Verification items for the finished model (mm, model axes). A direction names the side the tool comes from. Round coordinates to 2 decimals unless told otherwise and drop trailing zeros. Loops run counter-clockwise (first coordinate to the right, second up) from the corner with the lowest first, then second, coordinate; pieces in that order, holes last. Notation, with made-up numbers: (57.25, 70.5) - (104.25, 70.5) arc R18 cw to (104.25, 98.5) - close; hole circle Ø8 at (7.25, 76). An arc over 180 degrees is marked (long way). Use a Markdown table: item, result. Add a question column.
```python
from build123d import *

# Parameters (mm, degrees)
SKETCH1_W                    = 1165
SKETCH1_H                    = 40
BASE_FLANGE1_DEPTH           = 2
EDGE_FLANGE1_STRIP_W         = 13
EDGE_FLANGE1_STRIP_H         = 2
EDGE_FLANGE1_STRIP_CUT_DEPTH = 1165
EDGE_FLANGE1_DEPTH           = 1165
SKETCH9_R                    = 7.5
CUT_EXTRUDE1_DEPTH           = 671.102657441


# Sheet-metal steps are written as plain solids
with BuildPart() as part:
    # Sketch1 → Base-Flange1 (new body)
    with BuildSketch(Plane.XY):
        with Locations((-85.444287729, 62.85774027)):
            Rectangle(SKETCH1_W, SKETCH1_H)
        with BuildLine():
            Line((474.555712271, 57.85774027), (459.555712271, 57.85774027))
            ThreePointArc((459.555712271, 57.85774027), (454.555712271, 62.85774027), (459.555712271, 67.85774027))
            Line((459.555712271, 67.85774027), (474.555712271, 67.85774027))
            ThreePointArc((474.555712271, 67.85774027), (479.555712271, 62.85774027), (474.555712271, 57.85774027))
        make_face(mode=Mode.SUBTRACT)
        with BuildLine():
            Line((374.555712271, 57.85774027), (359.555712271, 57.85774027))
            ThreePointArc((359.555712271, 57.85774027), (354.555712271, 62.85774027), (359.555712271, 67.85774027))
            Line((359.555712271, 67.85774027), (374.555712271, 67.85774027))
            ThreePointArc((374.555712271, 67.85774027), (379.555712271, 62.85774027), (374.555712271, 57.85774027))
        make_face(mode=Mode.SUBTRACT)
    extrude(amount=-BASE_FLANGE1_DEPTH)

    # Edge-Flange1 strip (across the edge) → Edge-Flange1 strip cut (cut)
    with BuildSketch(Plane(origin=(497.055712271, 82.85774027, 0), x_dir=(0, -1, 0), z_dir=(-1, 0, 0))):
        with Locations((-2, -1)):
            Rectangle(EDGE_FLANGE1_STRIP_W, EDGE_FLANGE1_STRIP_H)
    extrude(amount=EDGE_FLANGE1_STRIP_CUT_DEPTH, mode=Mode.SUBTRACT)

    # Edge-Flange1 section (across the edge) → Edge-Flange1 (add)
    with BuildSketch(Plane(origin=(497.055712271, 82.85774027, 0), x_dir=(0, -1, 0), z_dir=(-1, 0, 0))):
        with BuildLine():
            Line((0, 2.5), (0, 38))
            Line((0, 38), (2, 38))
            Line((2, 38), (2, 2.5))
            ThreePointArc((2, 2.5), (2.732233047, 0.732233047), (4.5, 0))
            Line((4.5, 0), (4.5, -2))
            ThreePointArc((4.5, -2), (1.318019485, -0.681980515), (0, 2.5))
        make_face()
    extrude(amount=EDGE_FLANGE1_DEPTH)

    # Sketch9 → Cut-Extrude1 (cut, through all)
    with BuildSketch(Plane.XZ.offset(-80.85774027)):
        with Locations(Location((-647.944287729, 19, 0), (0, 0, 270))):
            Circle(SKETCH9_R)
        with Locations(Location((-567.944287729, 19, 0), (0, 0, 270))):
            Circle(SKETCH9_R)
    extrude(amount=-CUT_EXTRUDE1_DEPTH, mode=Mode.SUBTRACT)


solid = part.part
```
Q1. Go/stop test with flat-tipped pins: pin 1 Ø12 at (x, z) = (-567.94, 19) entering from +Y; pin 2 Ø1.6 at (x, z) = (466.5, -1) entering from +Y; pin 3 Ø17.5 at (x, y) = (-220, 52.5) entering from +Z; pin 4 Ø10.5 at (x, z) = (-193.5, 18) entering from -Y. Record where each tip stops, or that it passes through.
Q2. Section check B-B on x = -326.5. Record the cut outline in (y, z).
Q3. Section check C-C on y = 49. Record the cut outline in (x, z), plus the area to 3 significant figures.
Q4. Thickness scan on line 1 along X through (y, z) = (82, 19); line 2 along Y through (x, z) = (-434, 11); line 3 along Z through (x, y) = (15.5, 48). Record the ranges inside material, lowest first.
Q5. Set-up check for faces 1 (the face through (-77, 80.858, 20)), 2 (the face through (497.056, 82, 9)): record each of +Z, -Z, +X, -X, +Y, -Y from which the full face is reachable in a straight line by a thin tool's end or side.
Q6. Section check A-A on z = 19. Record the cut outline in (x, y), plus the area to 3 significant figures.
Determined:
| question | item | result |
|---|---|---|
| 1 | pin 1 | passes through |
| 1 | pin 2 | stops at y = 81.96 |
| 1 | pin 3 | stops at z = 0 |
| 1 | pin 4 | stops at y = 80.86 |
| 2 | outline | (42.86, -2) - (78.36, -2) arc R4.5 ccw to (82.86, 2.5) - (82.86, 38) - (80.86, 38) - (80.86, 2.5) arc R2.5 cw to (78.36, 0) - (42.86, 0) - close |
| 3 | outline | (-667.94, -2) - (497.06, -2) - (497.06, 0) - (-667.94, 0) - close |
| 3 | area | 2,330 mm² |
| 4 | line 1 | x = -667.94 to -655.44, -640.44 to -575.44, -560.44 to 497.06 |
| 4 | line 2 | y = 80.86 to 82.86 |
| 4 | line 3 | z = -2 to 0 |
| 5 | face 1 | +Z, +X, -X, -Y |
| 5 | face 2 | +Z, -Z, +X, +Y, -Y |
| 6 | outline | (-667.94, 80.86) - (-655.44, 80.86) - (-655.44, 82.86) - (-667.94, 82.86) - close; (-640.44, 80.86) - (-575.44, 80.86) - (-575.44, 82.86) - (-640.44, 82.86) - close; (-560.44, 80.86) - (497.06, 80.86) - (497.06, 82.86) - (-560.44, 82.86) - close |
| 6 | area | 2,270 mm² |
